from build123d import *

# Parameters (mm, degrees)
F1_DEPTH = 55
F2_R     = 1
F3_R     = 2.38125
F4_R     = 3.25
F5_DEPTH = 25
F6_SIZE  = 0.5


with BuildPart() as f1:
    # F0 (on Right) → F1 (new body, symmetric)
    with BuildSketch(Plane.YZ):
        Polygon((0, 25.4), (0, 0), (25.4, 0), (25.4, 4.7625), (4.7625, 4.7625), (4.7625, 25.4), align=None)
    extrude(amount=F1_DEPTH, both=True)

    # F2
    f2_edges = [f1.edges().sort_by_distance(p)[0] for p in [
        (0, 0, 25.4),
        (0, 4.7625, 25.4),
        (0, 0, 0),
        (0, 25.4, 4.7625),
        (0, 25.4, 0),
    ]]
    fillet(f2_edges, radius=F2_R)

    # F3
    f3_edges = [f1.edges().sort_by_distance(p)[0] for p in [
        (0, 4.7625, 4.7625),
    ]]
    fillet(f3_edges, radius=F3_R)

    # F4 (on face) → F5 (cut)
    with BuildSketch(Plane.XY.offset(4.7625)):
        with Locations((-40, 15)):
            Circle(F4_R)
        with Locations((690, 15)):
            Circle(F4_R)
        with Locations((1420, 15)):
            Circle(F4_R)
        with Locations((40, 15)):
            Circle(F4_R)
    extrude(amount=-F5_DEPTH, mode=Mode.SUBTRACT)

    # F6
    f6_edges = [f1.edges().sort_by_distance(p)[0] for p in [
        (-43.25, 15, 4.7625),
        (-36.75, 15, 2.38125),
        (-43.25, 15, 0),
        (36.75, 15, 4.7625),
        (43.25, 15, 2.38125),
        (36.75, 15, 0),
    ]]
    chamfer(f6_edges, length=F6_SIZE)


solid = f1.part
Can you work these out from the model? Positions are in its coordinate system, mm. A direction names the side the tool comes from. Give positions to 0.01 mm unless a question says otherwise; leave off trailing zeros. Order: outer loops, then holes, each group sorted by start corner. A loop starts at its lowest first (then second) coordinate and runs counter-clockwise, first axis right, second up. Notation, with made-up numbers: M 41.25,18.5 L 74.25,18.5 A13 ccw 74.25,38.5 Z; hole C -1.5,20.25 d6. An arc over 180 degrees is marked long. Use one line per item in the form item = value.
Item 1: If I drill on line 1 along Y through (x, z) = (-40, 3.2); line 2 along Z through (x, y) = (-32, 12), over which ranges is the centre line in solid material (lowest first)? Write a range as [from, to].
Values follow:
line_1 = [0, 11.75], [18.25, 25.4]
line_2 = [0, 4.76]
Item 2: If we section it at D-D, the plane z = 17.5: Write out the boundary of the cut face in (x, y), and give its area (3 significant figures).
Values follow:
outline = M -55,0 L 55,0 L 55,4.76 L -55,4.76 Z
area = 524 mm^2
Item 3: If we section it at C-C, the plane x = 2.5: Write out the boundary of the cut face in (y, z), and give its area (3 significant figures).
Values follow:
outline = M 0,1 A1 ccw 1,0 L 24.4,0 A1 ccw 25.4,1 L 25.4,3.76 A1 ccw 24.4,4.76 L 7.14,4.76 A2.38 cw 4.76,7.14 L 4.76,24.4 A1 ccw 3.76,25.4 L 1,25.4 A1 ccw 0,24.4 Z
area = 219 mm^2
Item 4: For faces 1 (the flat face through (1, 13, 0)), 2 (the flat face through (1, 16, 4.762)), which set-ups out of +Z, -Z, +X, -X, +Y, -Y let a thin tool reach every point of the face, with its end or its side?
Values follow:
face_1 = -Z, +X, -X, +Y, -Y
face_2 = +Z, +X, -X, +Y
Item 5: Thinking about a two-plate mould opening in X: for faces 3 (the cylindrical face through (43.1, 15.98, 2.41)), 4 (the flat face through (55, 4, 7)), 5 (the cylindrical face through (-0.77, 5.44, 5.48)), which applies, pulls with the +X half, pulls with the -X half, needs draft (parallel to the pull), parting line crosses it, or undercut?
Values follow:
face_3 = undercut
face_4 = pulls with the +X half
face_5 = needs draft
Item 6: Will these pins go through, and if not, where does the flat tip stop? pin 1 Ø8.5 at (x, y) = (40, 15) entering from +Z; pin 2 Ø5 at (x, z) = (16.5, 19) entering from +Y.
Values follow:
pin_1 = 4.76
pin_2 = 4.76
Item 7: If we section it at B-B, the plane y = 15: Write out the boundary of the cut face in (x, z), and give its area (3 significant figures).
Values follow:
outline = M -55,0 L -43.75,0 L -43.25,0.5 L -43.25,4.26 L -43.75,4.76 L -55,4.76 Z; M -36.75,0.5 L -36.25,0 L 36.25,0 L 36.75,0.5 L 36.75,4.26 L 36.25,4.76 L -36.25,4.76 L -36.75,4.26 Z; M 43.25,0.5 L 43.75,0 L 55,0 L 55,4.76 L 43.75,4.76 L 43.25,4.26 Z
area = 461 mm^2
Item 8: If we section it at A-A, the plane x = 40: Write out the boundary of the cut face in (y, z), and give its area (3 significant figures).
Values follow:
outline = M 0,1 A1 ccw 1,0 L 11.25,0 L 11.75,0.5 L 11.75,4.26 L 11.25,4.76 L 7.14,4.76 A2.38 cw 4.76,7.14 L 4.76,24.4 A1 ccw 3.76,25.4 L 1,25.4 A1 ccw 0,24.4 Z; M 18.25,0.5 L 18.75,0 L 24.4,0 A1 ccw 25.4,1 L 25.4,3.76 A1 ccw 24.4,4.76 L 18.75,4.76 L 18.25,4.26 Z
area = 188 mm^2
